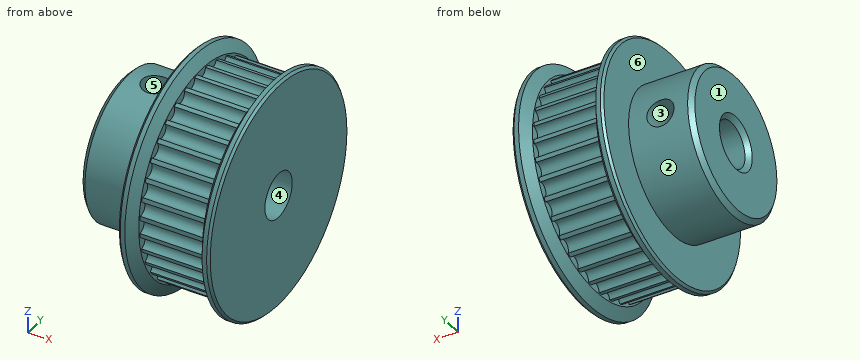
```python
from build123d import *

# Parameters (mm, degrees)
SCHIZZO5_R               = 0.75
TAGLIO_ESTRUSIONE1_DEPTH = 7
TAGLIO_ESTRUSIONE2_REACH = 14.75
SCHIZZO6_R               = 1.5
TAGLIO_ESTRUSIONE3_REACH = 14.75
SCHIZZO7_R               = 1.5
SMUSSO1_SIZE             = 0.5
SMUSSO2_SIZE             = 0.25


with BuildPart() as part:
    # Schizzo4 → Rivoluzione1 (revolve)
    with BuildSketch(Plane.XY):
        Polygon((0, 2.5), (0, 8), (7, 8), (7, 12.75), (7.75, 12.75), (8.5, 11.450961894), (8.5, 11.25), (15.5, 11.25), (15.5, 11.450961894), (16.25, 12.75), (17, 12.75), (17, 2.5), align=None)
    revolve(axis=Axis((0, 0, 0), (1, 0, 0)))

    # Schizzo5 → Taglio-Estrusione1 (cut)
    with BuildSketch(Plane(origin=(8.5, 0, 0), x_dir=(0, 0, -1), z_dir=(1, 0, 0))):
        with Locations((0, 11.25)):
            Circle(SCHIZZO5_R)
        with Locations((1.953541999, 11.079087221)):
            Circle(SCHIZZO5_R)
        with Locations((3.847726612, 10.571541984)):
            Circle(SCHIZZO5_R)
        with Locations((5.625, 9.742785793)):
            Circle(SCHIZZO5_R)
        with Locations((7.231360609, 8.617999985)):
            Circle(SCHIZZO5_R)
        with Locations((8.617999985, 7.231360609)):
            Circle(SCHIZZO5_R)
        with Locations((9.742785793, 5.625)):
            Circle(SCHIZZO5_R)
        with Locations((10.571541984, 3.847726612)):
            Circle(SCHIZZO5_R)
        with Locations((11.079087221, 1.953541999)):
            Circle(SCHIZZO5_R)
        with Locations((11.25, 0)):
            Circle(SCHIZZO5_R)
        with Locations((11.079087221, -1.953541999)):
            Circle(SCHIZZO5_R)
        with Locations((10.571541984, -3.847726612)):
            Circle(SCHIZZO5_R)
        with Locations((9.742785793, -5.625)):
            Circle(SCHIZZO5_R)
        with Locations((8.617999985, -7.231360609)):
            Circle(SCHIZZO5_R)
        with Locations((7.231360609, -8.617999985)):
            Circle(SCHIZZO5_R)
        with Locations((5.625, -9.742785793)):
            Circle(SCHIZZO5_R)
        with Locations((3.847726612, -10.571541984)):
            Circle(SCHIZZO5_R)
        with Locations((1.953541999, -11.079087221)):
            Circle(SCHIZZO5_R)
        with Locations((0, -11.25)):
            Circle(SCHIZZO5_R)
        with Locations((-1.953541999, -11.079087221)):
            Circle(SCHIZZO5_R)
        with Locations((-3.847726612, -10.571541984)):
            Circle(SCHIZZO5_R)
        with Locations((-5.625, -9.742785793)):
            Circle(SCHIZZO5_R)
        with Locations((-7.231360609, -8.617999985)):
            Circle(SCHIZZO5_R)
        with Locations((-8.617999985, -7.231360609)):
            Circle(SCHIZZO5_R)
        with Locations((-9.742785793, -5.625)):
            Circle(SCHIZZO5_R)
        with Locations((-10.571541984, -3.847726612)):
            Circle(SCHIZZO5_R)
        with Locations((-11.079087221, -1.953541999)):
            Circle(SCHIZZO5_R)
        with Locations((-11.25, 0)):
            Circle(SCHIZZO5_R)
        with Locations((-11.079087221, 1.953541999)):
            Circle(SCHIZZO5_R)
        with Locations((-10.571541984, 3.847726612)):
            Circle(SCHIZZO5_R)
        with Locations((-9.742785793, 5.625)):
            Circle(SCHIZZO5_R)
        with Locations((-8.617999985, 7.231360609)):
            Circle(SCHIZZO5_R)
        with Locations((-7.231360609, 8.617999985)):
            Circle(SCHIZZO5_R)
        with Locations((-5.625, 9.742785793)):
            Circle(SCHIZZO5_R)
        with Locations((-3.847726612, 10.571541984)):
            Circle(SCHIZZO5_R)
        with Locations((-1.953541999, 11.079087221)):
            Circle(SCHIZZO5_R)
    extrude(amount=TAGLIO_ESTRUSIONE1_DEPTH, mode=Mode.SUBTRACT)

    # Schizzo6 → Taglio-Estrusione2 (cut, up to next)
    with BuildSketch(Plane.XY, mode=Mode.PRIVATE) as taglio_estrusione2_sk1:
        with Locations((3.5, 0)):
            Circle(SCHIZZO6_R)
    taglio_estrusione2_tool1 = extrude(taglio_estrusione2_sk1.sketch, amount=TAGLIO_ESTRUSIONE2_REACH, mode=Mode.PRIVATE) & part.part
    add(taglio_estrusione2_tool1.solids().sort_by_distance((3.5, 0, 0))[0], mode=Mode.SUBTRACT)

    # Schizzo7 → Taglio-Estrusione3 (cut, up to next)
    with BuildSketch(Plane(origin=(0, 0, 0), x_dir=(1, 0, 0), z_dir=(0, 1, 0)), mode=Mode.PRIVATE) as taglio_estrusione3_sk1:
        with Locations((3.5, 0)):
            Circle(SCHIZZO7_R)
    taglio_estrusione3_tool1 = extrude(taglio_estrusione3_sk1.sketch, amount=TAGLIO_ESTRUSIONE3_REACH, mode=Mode.PRIVATE) & part.part
    add(taglio_estrusione3_tool1.solids().sort_by_distance((3.5, 0, 0))[0], mode=Mode.SUBTRACT)

    # Smusso1
    smusso1_edges = [part.edges().sort_by_distance(p)[0] for p in [
        (0, -8, 0),
        (0, -2.5, 0),
    ]]
    chamfer(smusso1_edges, length=SMUSSO1_SIZE)

    # Smusso2
    smusso2_edges = [part.edges().sort_by_distance(p)[0] for p in [
        (7, -12.75, 0),
        (17, -12.75, 0),
    ]]
    chamfer(smusso2_edges, length=SMUSSO2_SIZE)


solid = part.part
```
CAD build for the part. Positions are in the model's coordinates, mm. Face numbers are marked on the shaded views. A direction names the side the tool comes from. Give positions to 0.01 mm unless a question says otherwise; leave off trailing zeros. Order: outer loops, then holes, each group sorted by start corner. A loop starts at its lowest first (then second) coordinate and runs counter-clockwise, first axis right, second up.
(1) Flat gauge pins, fed straight in: pin 1 (4 mm diameter, centred on x = 3.5, y = 0, fed in from -Z); pin 2 (1.5 mm diameter, centred on x = 12, z = 2.5, fed in from -Y); pin 3 (4 mm diameter, centred on x = 2.5, z = -9, fed in from -Y); pin 4 (7 mm diameter, centred on y = -2.5, z = -4, fed in from -X). Where does each tip first touch, or does it go through?
(2) Drill centre lines: L1, parallel to Z at x = 9, y = 0; L2, parallel to X at y = 0, z = 3; L3, parallel to Y at x = 13.5, z = 2. Where is each one in solid material? Low to high.
(3) Saw through at B-B, the plane z = 0. State how many separate pieces and enclosed holes the cut face has, then the cut area to 3 significant figures.
(4) Tool access for the marked faces 4, 5 and 6: list every direction of +Z, -Z, +X, -X, +Y, -Y with a clear straight run to the whole face (end or side of a thin tool).
(5) Mould opens along Z. For the marked faces 1, 2 and 3 say: released by +Z, released by -Z, zero draft, split by the parting line, or undercut.
(6) Saw through at A-A, the plane x = 3. Give the cut face in (y, z).
Results found:
1. pin 1: stops at z = -8
1. pin 2: stops at y = -10.92
1. pin 3: stops at y = -3.87
1. pin 4: stops at x = 0
2. L1: z = -10.5 to -2.5, 2.5 to 10.5
2. L2: x = 0 to 2, 5 to 17
2. L3: y = -10.33 to -1.5, 1.5 to 10.33
3. separate pieces: 3
3. enclosed holes: 0
3. area: 231 mm2
4. face 4: +X, -X
4. face 5: +Z
4. face 6: -X
5. face 1: zero draft
5. face 2: split by the parting line
5. face 3: undercut
6. outline: (-1.41, 2.06) - (-1.41, 7.87) arc R8 ccw (long way) to (7.87, -1.41) - (2.06, -1.41) arc R2.5 cw (long way) to start; (1.41, 2.06) arc R2.5 cw to (2.06, 1.41) - (7.87, 1.41) arc R8 ccw to (1.41, 7.87) - close
